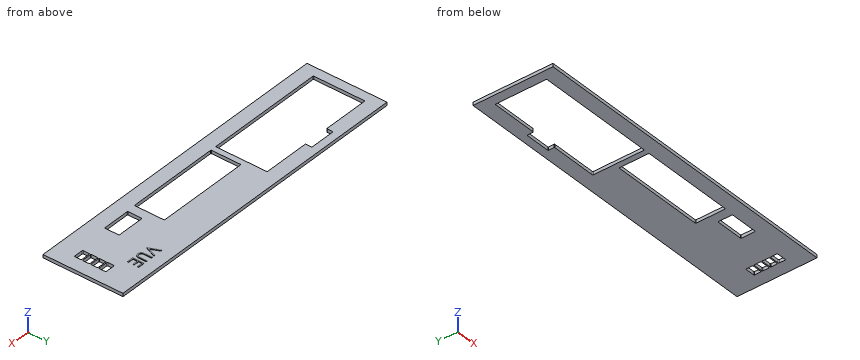
from build123d import *

# Parameters (mm, degrees)
ESQUISSE1_W             = 100
ESQUISSE1_H             = 24.8
BOSS_EXTRU_1_DEPTH      = 1
ESQUISSE2_W             = 29
ESQUISSE2_H             = 9.3
ESQUISSE2_W_2           = 8.7
ESQUISSE2_H_2           = 4.5
ESQUISSE2_W_3           = 3.2
ESQUISSE2_H_3           = 2.2
ENL_V_MAT_EXTRU_1_DEPTH = 52.524363169
CONG_1_R                = 0.2
BOSS_EXTRU_2_DEPTH      = 0.1


with BuildPart() as part:
    # Esquisse1 → Boss.-Extru.1 (new body)
    with BuildSketch(Plane.XY):
        Rectangle(ESQUISSE1_W, ESQUISSE1_H)
    extrude(amount=BOSS_EXTRU_1_DEPTH)

    # Esquisse2 → Enlèv. mat.-Extru.1 (cut, through all)
    with BuildSketch(Plane.XY.offset(1)):
        Polygon((-47.0074, 8), (-32.5074, 8), (-32.5074, 10), (-24.5074, 10), (-24.5074, 8), (-10.0074, 8), (-10.0074, -8), (-47.0074, -8), align=None)
        with Locations((6.25, -3.35)):
            Rectangle(ESQUISSE2_W, ESQUISSE2_H)
        with Locations((28, -5.5)):
            Rectangle(ESQUISSE2_W_2, ESQUISSE2_H_2)
        with Locations((44.255985376, 2.61)):
            Rectangle(ESQUISSE2_W_3, ESQUISSE2_H_3)
        with Locations((44.255985376, 0.07)):
            Rectangle(ESQUISSE2_W_3, ESQUISSE2_H_3)
        with Locations((44.255985376, -2.47)):
            Rectangle(ESQUISSE2_W_3, ESQUISSE2_H_3)
        with Locations((44.255985376, -5.01)):
            Rectangle(ESQUISSE2_W_3, ESQUISSE2_H_3)
    extrude(amount=-ENL_V_MAT_EXTRU_1_DEPTH, mode=Mode.SUBTRACT)

    # Congé1
    cong_1_edges = [part.edges().sort_by_distance(p)[0] for p in [
        (45.855985376, -3.91, 0.5),
        (45.855985376, -6.11, 0.5),
        (42.655985376, -6.11, 0.5),
        (42.655985376, -3.91, 0.5),
        (-47.0074, -8, 0.5),
        (-47.0074, 8, 0.5),
        (-32.5074, 8, 0.5),
        (-32.5074, 10, 0.5),
        (-24.5074, 10, 0.5),
        (-24.5074, 8, 0.5),
        (-10.0074, 8, 0.5),
        (-10.0074, -8, 0.5),
        (-8.25, -8, 0.5),
        (-8.25, 1.3, 0.5),
        (20.75, 1.3, 0.5),
        (20.75, -8, 0.5),
        (23.65, -7.75, 0.5),
        (23.65, -3.25, 0.5),
        (32.35, -3.25, 0.5),
        (32.35, -7.75, 0.5),
        (45.855985376, 3.71, 0.5),
        (45.855985376, 1.51, 0.5),
        (42.655985376, 1.51, 0.5),
        (42.655985376, 3.71, 0.5),
        (45.855985376, 1.17, 0.5),
        (45.855985376, -1.03, 0.5),
        (42.655985376, -1.03, 0.5),
        (42.655985376, 1.17, 0.5),
        (45.855985376, -1.37, 0.5),
        (45.855985376, -3.57, 0.5),
        (42.655985376, -3.57, 0.5),
        (42.655985376, -1.37, 0.5),
    ]]
    fillet(cong_1_edges, radius=CONG_1_R)

    # Esquisse3 → Boss.-Extru.2 (add)
    with BuildSketch(Plane.XY.offset(1)):
        Polygon((30.691975839, 8.654898364), (31.028514301, 8.654898364), (32.195180967, 5.896685223), (33.361847634, 8.654898364), (33.698386096, 8.654898364), (32.217616865, 5.154898364), (32.17274507, 5.154898364), align=None)
        with BuildLine():
            Line((34.326591224, 8.654898364), (34.640693788, 8.654898364))
            Line((34.640693788, 8.654898364), (34.640693788, 6.557843075))
            add(Edge.make_bspline(
                [(34.640693788, 6.557843075), (34.640647044, 6.528162339), (34.640558339, 6.471838028), (34.641150853, 6.391669728), (34.642810222, 6.320397269), (34.643856381, 6.257745921), (34.646183715, 6.204003174), (34.648081761, 6.158877863), (34.650522318, 6.122583661), (34.653455436, 6.101402735), (34.654716224, 6.092298203)],
                knots=[0, 0, 0, 0, 1.528628734, 2.90083645, 4.128790002, 5.200304208, 6.127813768, 6.898992206, 7.526736466, 8, 8, 8, 8], degree=3))
            add(Edge.make_bspline(
                [(34.654716224, 6.092298203), (34.659893683, 6.05945144), (34.669956869, 5.995608711), (34.695603247, 5.904700429), (34.731420748, 5.822768971), (34.77386379, 5.74725768), (34.829796402, 5.68026832), (34.896799937, 5.618556667), (34.977977706, 5.564584862), (35.068238311, 5.51523405), (35.165523549, 5.475568968), (35.264934815, 5.445575604), (35.364977794, 5.427296704), (35.431953959, 5.425180165), (35.465213019, 5.424129133)],
                knots=[0, 0, 0, 0, 1.035780045, 2.013197591, 2.933192213, 3.817615948, 4.702609284, 5.640816605, 6.646850145, 7.73207398, 8.84249596, 9.914020372, 10.964143139, 12, 12, 12, 12], degree=3))
            add(Edge.make_bspline(
                [(35.465213019, 5.424129133), (35.493766759, 5.425202983), (35.550709321, 5.427344481), (35.635315752, 5.440605912), (35.71771586, 5.464506478), (35.79831654, 5.495346237), (35.873867525, 5.536093828), (35.944410967, 5.583164667), (36.007374901, 5.638375543), (36.064832899, 5.699475888), (36.114867835, 5.768415688), (36.158238976, 5.843693826), (36.193764906, 5.926443173), (36.211308431, 5.984597595), (36.220321192, 6.014473684)],
                knots=[0, 0, 0, 0, 0.994687771, 1.983630487, 2.973142513, 3.978332533, 4.983357753, 5.956394766, 6.925816176, 7.893390482, 8.871859704, 9.88551698, 10.913711441, 12, 12, 12, 12], degree=3))
            add(Edge.make_bspline(
                [(36.220321192, 6.014473684), (36.223321317, 6.026822258), (36.230006805, 6.054339859), (36.23625385, 6.100861149), (36.242760376, 6.155750513), (36.247274946, 6.219402326), (36.251676166, 6.291603299), (36.254309239, 6.372729556), (36.255526272, 6.462486517), (36.255888952, 6.525123679), (36.256078403, 6.557843075)],
                knots=[0, 0, 0, 0, 0.558680831, 1.244966039, 2.062412453, 2.990489873, 4.051219941, 5.244515665, 6.560634259, 8, 8, 8, 8], degree=3))
            Line((36.256078403, 6.557843075), (36.256078403, 8.654898364))
            Line((36.256078403, 8.654898364), (36.570180967, 8.654898364))
            Line((36.570180967, 8.654898364), (36.570180967, 6.541016152))
            add(Edge.make_bspline(
                [(36.570180967, 6.541016152), (36.569926847, 6.502917773), (36.569430916, 6.42856647), (36.565130339, 6.319615111), (36.558273339, 6.21626213), (36.548585251, 6.118493633), (36.535748248, 6.026659474), (36.521473028, 5.939954706), (36.503293495, 5.859001713), (36.482060093, 5.783169296), (36.457786545, 5.710983782), (36.426345397, 5.642475168), (36.390920897, 5.575560768), (36.348906244, 5.511252659), (36.301694862, 5.449266106), (36.248243181, 5.389977031), (36.19031902, 5.332437985), (36.12695946, 5.278124919), (36.059208935, 5.228316242), (35.987268977, 5.184518471), (35.911692208, 5.147494853), (35.832675082, 5.117018929), (35.750183879, 5.094104329), (35.664216519, 5.077029174), (35.574577326, 5.067326876), (35.513612669, 5.065884946), (35.482741064, 5.065154774)],
                knots=[0, 0, 0, 0, 1.316592851, 2.569410997, 3.76748051, 4.895814652, 5.963796859, 6.97159953, 7.931736103, 8.829262218, 9.692595152, 10.560224239, 11.431080259, 12.30701507, 13.211635791, 14.121146779, 15.063487852, 16.031507147, 17.00238618, 17.966455255, 18.938106653, 19.907068911, 20.888905087, 21.893141452, 22.933117798, 24, 24, 24, 24], degree=3))
            add(Edge.make_bspline(
                [(35.482741064, 5.065154774), (35.449071961, 5.065939539), (35.383013302, 5.067479246), (35.285675235, 5.076301996), (35.192361039, 5.09292039), (35.102085161, 5.114080334), (35.016076664, 5.143264071), (34.93318322, 5.177362196), (34.854824539, 5.219239456), (34.77972941, 5.265832849), (34.709904654, 5.318257488), (34.645807251, 5.375397662), (34.58733138, 5.436338039), (34.535462684, 5.501738405), (34.489341799, 5.571090112), (34.449611586, 5.644589352), (34.415498342, 5.722207668), (34.397891775, 5.776160868), (34.388991064, 5.803436024)],
                knots=[0, 0, 0, 0, 1.13879206, 2.234305948, 3.301075583, 4.341971843, 5.366689343, 6.369221514, 7.369726634, 8.367512178, 9.355451585, 10.318319045, 11.268648973, 12.207971039, 13.137398894, 14.081662264, 15.030215811, 16, 16, 16, 16], degree=3))
            add(Edge.make_bspline(
                [(34.388991064, 5.803436024), (34.383813905, 5.822068598), (34.372584534, 5.862483067), (34.360559236, 5.929369556), (34.350450155, 6.006384473), (34.340944597, 6.093533092), (34.335335639, 6.190882958), (34.3304182, 6.298391874), (34.326556581, 6.416189836), (34.326579353, 6.498244352), (34.326591224, 6.541016152)],
                knots=[0, 0, 0, 0, 0.625038921, 1.35572334, 2.194682327, 3.136881307, 4.189498639, 5.346923369, 6.617055217, 8, 8, 8, 8], degree=3))
            Line((34.326591224, 6.541016152), (34.326591224, 8.654898364))
        make_face()
        Polygon((37.467616865, 8.654898364), (39.441975839, 8.654898364), (39.441975839, 8.295924005), (37.781719429, 8.295924005), (37.781719429, 7.219000928), (39.441975839, 7.219000928), (39.441975839, 6.860026569), (37.781719429, 6.860026569), (37.781719429, 5.513872723), (39.441975839, 5.513872723), (39.441975839, 5.154898364), (37.467616865, 5.154898364), align=None)
    extrude(amount=BOSS_EXTRU_2_DEPTH)


solid = part.part
Part model, mm, in its own coordinate system. Coordinates: 2 decimals unless noted, no trailing zeros. Write each loop counter-clockwise with the first axis right and the second up, starting at its lowest first coordinate (ties: lowest second). Pieces come first, ordered by that corner, then holes. Notation, with made-up numbers: M 62.5,46.25 L 90.5,46.25 A8 ccw 90.5,56.25 Z; hole C -23.75,-19.75 d1. An arc over 180 degrees is marked long. Return JSON: item names as keys, results as strings.
1. Saw through at B-B, the plane x = 2. Write the cut outline in (y, z).
Determined:
{"outline": "M -12.4,0 L -8,0 L -8,1 L -12.4,1 Z; M 1.3,0 L 12.4,0 L 12.4,1 L 1.3,1 Z"}
2. Probe L1, parallel to X at y = 2, z = 0.55; L2, parallel to X at y = -5.75, z = 0.9; L3, parallel to X at y = -3.75, z = 0.2. List the from-to ranges inside material, lowest first.
Determined:
{"L1": "-50 to -47.01, -10.01 to 42.66, 45.86 to 50", "L2": "-50 to -47.01, -10.01 to -8.25, 20.75 to 23.65, 32.35 to 42.66, 45.86 to 50", "L3": "-50 to -47.01, -10.01 to -8.25, 20.75 to 23.65, 32.35 to 50"}
3. Flat gauge pin, fed straight in: pin 1 Ø6 at (x, y) = (15.5, -3) entering from -Z. Where does the tip first touch, or does it go through?
Determined:
{"pin 1": "through"}
4. Saw through at C-C, the plane z = 0.2. Count the separate pieces of the cut face and the enclosed holes in it, then the cut area to 3 significant figures.
Determined:
{"separate pieces": "1", "enclosed holes": "7", "area": "1,540 mm²"}
5. Saw through at D-D, the plane y = -10.25. Write the cut outline in (x, z), then the cut area to 3 significant figures.
Determined:
{"outline": "M -50,0 L 50,0 L 50,1 L -50,1 Z", "area": "100 mm²"}
6. Saw through at A-A, the plane x = -28. Write the cut outline in (y, z), then the cut area to 3 significant figures.
Determined:
{"outline": "M -12.4,0 L -8,0 L -8,1 L -12.4,1 Z; M 10,0 L 12.4,0 L 12.4,1 L 10,1 Z", "area": "6.80 mm²"}
